```python
from build123d import *

# Parameters (mm, degrees)
F0_W     = 12
F0_H     = 4.5
F1_DEPTH = 15
F2_W     = 2
F2_H     = 2
F3_DEPTH = 3


with BuildPart() as f1:
    # F0 (on Top) → F1 (new body)
    with BuildSketch(Plane.XY):
        with Locations((6, 2.25)):
            Rectangle(F0_W, F0_H)
    extrude(amount=F1_DEPTH)

    # F2 (on face) → F3 (cut)
    with BuildSketch(Plane.XZ):
        with Locations((3, 12)):
            Rectangle(F2_W, F2_H)
        with Locations((6.2, 12)):
            Rectangle(F2_W, F2_H)
        with Locations((9.4, 12)):
            Rectangle(F2_W, F2_H)
        with Locations((2.98, 8.26)):
            Rectangle(F2_W, F2_H)
        with Locations((6.18, 8.26)):
            Rectangle(F2_W, F2_H)
        with Locations((9.38, 8.26)):
            Rectangle(F2_W, F2_H)
        with Locations((2.96, 4.52)):
            Rectangle(F2_W, F2_H)
        with Locations((6.16, 4.52)):
            Rectangle(F2_W, F2_H)
        with Locations((9.36, 4.52)):
            Rectangle(F2_W, F2_H)
    extrude(amount=-F3_DEPTH, mode=Mode.SUBTRACT)


solid = f1.part
```
CAD build for the part. Positions are in the model's coordinates, mm. A direction names the side the tool comes from. Coordinates: 2 decimals unless noted, no trailing zeros. Write each loop counter-clockwise with the first axis right and the second up, starting at its lowest first coordinate (ties: lowest second). Pieces come first, ordered by that corner, then holes. Notation, with made-up numbers: (80.25, 56.5) -> (117.25, 56.5) arc R29 cw to (117.25, 86.5) -> close; hole circle Ø5 at (75, 48.5). An arc over 180 degrees is marked (long way). Return JSON: item names as keys, results as strings. Group by question number.
Q1. Cut at A-A, the plane x = 6.5. Give the cut face in (y, z), then the cut area to 3 significant figures.
Q2. Cut at C-C, the plane y = 0.5. State how many separate pieces and enclosed holes the cut face has, then the cut area to 3 significant figures.
Q3. Flat gauge pins, fed straight in: pin 1 (3 mm diameter, centred on x = 10, z = 7.5, fed in from -Y); pin 2 (0.6 mm diameter, centred on x = 6.5, z = 8, fed in from -Y). Where does each tip first touch, or does it go through?
Q4. Cut at B-B, the plane z = 3.75. Give the cut face in (x, y), then the cut area to 3 significant figures.
Q5. Pull direction Z, two halves, no side cores. Call faces 1 (the face through (5.16, 1, 5)), 2 (the face through (6, 2, 15)), 3 (the face through (6, 4.5, 7)), 4 (the face through (1.96, 1, 5)): released by +Z, released by -Z, zero draft, split by the parting line, or undercut.
Q6. Which spindle directions (+Z, -Z, +X, -X, +Y, -Y) get a long thin tool onto all of the face, cutting with end or side? Do faces 5 (the face through (0, 2, 7)), 6 (the face through (6, 1, 9.26)). Say none if no direction does.
Q7. Drill centre lines: line 1 (X direction, y = 2.7, z = 5); line 2 (Z direction, x = 8.5, y = 2.7); line 3 (Y direction, x = 3.25, z = 4). Where is each one in solid material? Low to high.
Returned:
{
 "1": {"outline": "(0, 0) -> (4.5, 0) -> (4.5, 15) -> (0, 15) -> (0, 13) -> (3, 13) -> (3, 11) -> (0, 11) -> (0, 9.26) -> (3, 9.26) -> (3, 7.26) -> (0, 7.26) -> (0, 5.52) -> (3, 5.52) -> (3, 3.52) -> (0, 3.52) -> close", "area": "49.5 mm2"},
 "2": {"separate pieces": "1", "enclosed holes": "9", "area": "144 mm2"},
 "3": {"pin 1": "stops at y = 0", "pin 2": "stops at y = 3"},
 "4": {"outline": "(0, 0) -> (1.96, 0) -> (1.96, 3) -> (3.96, 3) -> (3.96, 0) -> (5.16, 0) -> (5.16, 3) -> (7.16, 3) -> (7.16, 0) -> (8.36, 0) -> (8.36, 3) -> (10.36, 3) -> (10.36, 0) -> (12, 0) -> (12, 4.5) -> (0, 4.5) -> close", "area": "36.0 mm2"},
 "5": {"face 1": "undercut", "face 2": "released by +Z", "face 3": "zero draft", "face 4": "undercut"},
 "6": {"face 5": "+Z, -Z, -X, +Y, -Y", "face 6": "-Y"},
 "7": {"line 1": "x = 0 to 1.96, 3.96 to 5.16, 7.16 to 8.36, 10.36 to 12", "line 2": "z = 0 to 3.52, 5.52 to 7.26, 9.26 to 11, 13 to 15", "line 3": "y = 3 to 4.5"}
}
